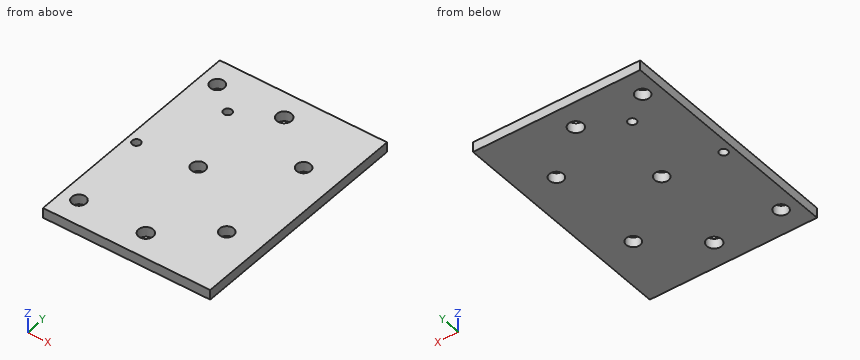
from build123d import *

# Parameters (mm, degrees)
SKETCH_1_W          = 40
SKETCH_1_H          = 29
EXTRUDE_1_DEPTH     = 3
SKETCH_3_W          = 40
SKETCH_3_H          = 3
EXTRUDE_2_DEPTH     = 3
SKETCH_4_W          = 40
SKETCH_4_H          = 3
EXTRUDE_3_DEPTH     = 3
SKETCH_5_W          = 40
SKETCH_5_H          = 3
EXTRUDE_4_DEPTH     = 7
SKETCH_6_W          = 40
SKETCH_6_H          = 3
EXTRUDE_5_DEPTH     = 7
SKETCH_7_W          = 40
SKETCH_7_H          = 3
EXTRUDE_6_DEPTH     = 10
SKETCH_8_W          = 40
SKETCH_8_H          = 3
EXTRUDE_7_DEPTH     = 10
SKETCH_9_R          = 2.2
CUT_EXTRUDE_2_DEPTH = 15
CUT_EXTRUDE_3_DEPTH = 4
SKETCH_12_W         = 3
SKETCH_12_H         = 69
EXTRUDE_9_DEPTH     = 30
SKETCH_15_R         = 2.1
CUT_EXTRUDE_4_DEPTH = 10
SKETCH_16_R         = 2.1
CUT_EXTRUDE_5_DEPTH = 10
SKETCH_17_W         = 3
SKETCH_17_H         = 69
CUT_EXTRUDE_6_DEPTH = 20
M3X0_5_1_D          = 2.5
M3X0_5_1_DEPTH      = 8.5
M3X0_5_1_TIP        = 0.751075774
SKETCH_20_R         = 2.1
CUT_EXTRUDE_7_DEPTH = 10


with BuildPart() as part:
    # ｽｹｯﾁ1 → ﾎﾞｽ - 押し出し1 (new body)
    with BuildSketch(Plane.XY):
        Rectangle(SKETCH_1_W, SKETCH_1_H)
    extrude(amount=EXTRUDE_1_DEPTH)

    # ｽｹｯﾁ3 → ﾎﾞｽ - 押し出し2 (add)
    with BuildSketch(Plane(origin=(0, -14.5, 0), x_dir=(-1, 0, 0), z_dir=(0, -1, 0))):
        with Locations((0, -1.5)):
            Rectangle(SKETCH_3_W, SKETCH_3_H)
    extrude(amount=EXTRUDE_2_DEPTH)

    # ｽｹｯﾁ4 → ﾎﾞｽ - 押し出し3 (add)
    with BuildSketch(Plane(origin=(0, 14.5, 0), x_dir=(1, 0, 0), z_dir=(0, 1, 0))):
        with Locations((0, -1.5)):
            Rectangle(SKETCH_4_W, SKETCH_4_H)
    extrude(amount=EXTRUDE_3_DEPTH)

    # ｽｹｯﾁ5 → ﾎﾞｽ - 押し出し4 (add)
    with BuildSketch(Plane.XZ.offset(17.5)):
        with Locations((0, 1.5)):
            Rectangle(SKETCH_5_W, SKETCH_5_H)
    extrude(amount=EXTRUDE_4_DEPTH)

    # ｽｹｯﾁ6 → ﾎﾞｽ - 押し出し5 (add)
    with BuildSketch(Plane(origin=(0, 17.5, 0), x_dir=(1, 0, 0), z_dir=(0, 1, 0))):
        with Locations((0, -1.5)):
            Rectangle(SKETCH_6_W, SKETCH_6_H)
    extrude(amount=EXTRUDE_5_DEPTH)

    # ｽｹｯﾁ7 → ﾎﾞｽ - 押し出し6 (add)
    with BuildSketch(Plane(origin=(0, 24.5, 0), x_dir=(1, 0, 0), z_dir=(0, 1, 0))):
        with Locations((0, -1.5)):
            Rectangle(SKETCH_7_W, SKETCH_7_H)
    extrude(amount=EXTRUDE_6_DEPTH)

    # ｽｹｯﾁ8 → ﾎﾞｽ - 押し出し7 (add)
    with BuildSketch(Plane.XZ.offset(24.5)):
        with Locations((0, 1.5)):
            Rectangle(SKETCH_8_W, SKETCH_8_H)
    extrude(amount=EXTRUDE_7_DEPTH)

    # ｽｹｯﾁ9 → ｶｯﾄ - 押し出し2 (cut)
    with BuildSketch(Plane.XY.offset(3)):
        with Locations((-5, 27)):
            Circle(SKETCH_9_R)
    extrude(amount=-CUT_EXTRUDE_2_DEPTH, mode=Mode.SUBTRACT)

    # ｽｹｯﾁ10 → ｶｯﾄ - 押し出し3 (cut, through all)
    with BuildSketch(Plane.XY.offset(3)):
        with BuildLine():
            ThreePointArc((-7.2, -27), (-5, -29.2), (-2.8, -27))
            Line((-2.8, -27), (-5, -27))
            Line((-5, -27), (-7.2, -27))
        make_face()
        with BuildLine():
            Line((-5, -27), (-2.8, -27))
            ThreePointArc((-2.8, -27), (-5, -24.8), (-7.2, -27))
            Line((-7.2, -27), (-5, -27))
        make_face()
    extrude(amount=-CUT_EXTRUDE_3_DEPTH, mode=Mode.SUBTRACT)

    # ｽｹｯﾁ12 → ﾎﾞｽ - 押し出し9 (add)
    with BuildSketch(Plane.ZY.offset(20)):
        with Locations((1.5, 0)):
            Rectangle(SKETCH_12_W, SKETCH_12_H)
    extrude(amount=EXTRUDE_9_DEPTH)

    # ｽｹｯﾁ15 → ｶｯﾄ - 押し出し4 (cut)
    with BuildSketch(Plane.XY.offset(3)):
        with Locations((-10, 0)):
            Circle(SKETCH_15_R)
    extrude(amount=-CUT_EXTRUDE_4_DEPTH, mode=Mode.SUBTRACT)

    # ｽｹｯﾁ16 → ｶｯﾄ - 押し出し5 (cut)
    with BuildSketch(Plane(origin=(0, 0, 0), x_dir=(-1, 0, 0), z_dir=(0, 0, -1))):
        with Locations((-10, -15)):
            Circle(SKETCH_16_R)
        with Locations((-10, 15)):
            Circle(SKETCH_16_R)
    extrude(amount=-CUT_EXTRUDE_5_DEPTH, mode=Mode.SUBTRACT)

    # ｽｹｯﾁ17 → ｶｯﾄ - 押し出し6 (cut)
    with BuildSketch(Plane.ZY.offset(50)):
        with Locations((1.5, 0)):
            Rectangle(SKETCH_17_W, SKETCH_17_H)
    extrude(amount=-CUT_EXTRUDE_6_DEPTH, mode=Mode.SUBTRACT)

    # M3x0.5 ねじ穴1
    with Locations(Plane(origin=(-16.881888018, 20.463438375, 3), x_dir=(1, 0, 0), z_dir=(0, 0, 1))):
        with Locations((0, 0), (-10.3, -22.2)):
            Hole(M3X0_5_1_D / 2, depth=M3X0_5_1_DEPTH)
            with Locations((0, 0, -(M3X0_5_1_DEPTH + M3X0_5_1_TIP / 2))):  # 118° drill point
                Cone(0, M3X0_5_1_D / 2, M3X0_5_1_TIP, mode=Mode.SUBTRACT)

    # ｽｹｯﾁ20 → ｶｯﾄ - 押し出し7 (cut)
    with BuildSketch(Plane(origin=(0, 0, 0), x_dir=(-1, 0, 0), z_dir=(0, 0, -1))):
        with Locations((25, -27)):
            Circle(SKETCH_20_R)
        with Locations((25, 27)):
            Circle(SKETCH_20_R)
    extrude(amount=-CUT_EXTRUDE_7_DEPTH, mode=Mode.SUBTRACT)


solid = part.part
Could you check a few things on this model? Use its own coordinates, in mm. Coordinates: 2 decimals unless noted, no trailing zeros. Order: outer loops, then holes, each group sorted by start corner. A loop starts at its lowest first (then second) coordinate and runs counter-clockwise, first axis right, second up.
Q1. Suppose I cut it at B-B on x = 10. Please give me the cut outline in (y, z).
Q2. Suppose I cut it at C-C on y = -27. Please give me the cut outline in (x, z), and give its area (3 significant figures).
Q3. Suppose I cut it at A-A on y = -15. Please give me the cut outline in (x, z), and give its area (3 significant figures).
Q4. Will this pin go through, and if not, where does the flat tip stop? pin 1 (1.5 mm diameter, centred on x = -27.18, y = -1.74, fed in from -Z).
Q5. Please list where these lines run through material, in increasing order: L1, parallel to Y at x = -5, z = 0.75; L2, parallel to Y at x = -25, z = 1.5; L3, parallel to Y at x = -10, z = 2.5.
Q6. Suppose I cut it at D-D on x = -10. Please give me the cut outline in (y, z), and give its area (3 significant figures).
Answer:
1. outline: (-34.5, 0) - (-17.1, 0) - (-17.1, 3) - (-34.5, 3) - close; (-12.9, 0) - (12.9, 0) - (12.9, 3) - (-12.9, 3) - close; (17.1, 0) - (34.5, 0) - (34.5, 3) - (17.1, 3) - close
2. outline: (-30, 0) - (-27.1, 0) - (-27.1, 3) - (-30, 3) - close; (-22.9, 0) - (-7.2, 0) - (-7.2, 3) - (-22.9, 3) - close; (-2.8, 0) - (20, 0) - (20, 3) - (-2.8, 3) - close
2. area: 124 mm2
3. outline: (-30, 0) - (7.9, 0) - (7.9, 3) - (-30, 3) - close; (12.1, 0) - (20, 0) - (20, 3) - (12.1, 3) - close
3. area: 137 mm2
4. pin 1: passes through
5. L1: y = -34.5 to -29.2, -24.8 to 24.8, 29.2 to 34.5
5. L2: y = -34.5 to -29.1, -24.9 to 24.9, 29.1 to 34.5
5. L3: y = -34.5 to -2.1, 2.1 to 34.5
6. outline: (-34.5, 0) - (-2.1, 0) - (-2.1, 3) - (-34.5, 3) - close; (2.1, 0) - (34.5, 0) - (34.5, 3) - (2.1, 3) - close
6. area: 194 mm2
